from build123d import *

# Parameters (mm, degrees)
SKETCH1_R           = 14
SKETCH1_R_2         = 9
BOSS_EXTRUDE1_DEPTH = 17.5
SKETCH5_R           = 9.5
SKETCH5_R_2         = 7
BOSS_EXTRUDE2_DEPTH = 9.5
BOSS_EXTRUDE3_DEPTH = 2.5
SKETCH7_W           = 5
SKETCH7_H           = 17.5
BOSS_EXTRUDE4_DEPTH = 0.225023
BOSS_EXTRUDE5_DEPTH = 2.5
BOSS_EXTRUDE9_DEPTH = 2.5


with BuildPart() as part:
    # Sketch1 → Boss-Extrude1 (new, symmetric)
    with BuildSketch(Plane.XY):
        Circle(SKETCH1_R)
        Circle(SKETCH1_R_2, mode=Mode.SUBTRACT)
    extrude(amount=BOSS_EXTRUDE1_DEPTH, both=True)



with BuildPart() as body_2:
    # Sketch5 → Boss-Extrude2 (new, symmetric)
    with BuildSketch(Plane(origin=(0, 0, 0), x_dir=(0, 0, -1), z_dir=(1, 0, 0))):
        with Locations((0, 26)):
            Circle(SKETCH5_R)
        with Locations((0, 26)):
            Circle(SKETCH5_R_2, mode=Mode.SUBTRACT)
    extrude(amount=BOSS_EXTRUDE2_DEPTH, both=True)

    # Sketch6 → Boss-Extrude3 (add, symmetric)
    with BuildSketch(Plane(origin=(0, 0, 0), x_dir=(0, 0, -1), z_dir=(1, 0, 0))):
        with BuildLine():
            Line((-8.311766618, 30.600492984), (-17.5, 14))
            Line((-17.5, 14), (0, 14))
            Line((0, 14), (0, 16.5))
            ThreePointArc((0, 16.5), (-8.183968577, 21.175825633), (-8.311766618, 30.600492984))
        make_face()
    extrude(amount=BOSS_EXTRUDE3_DEPTH, both=True)


with BuildPart() as part_1:
    add(part.part)

    add(body_2.part)  # Boss-Extrude4 merges body 2
    # Sketch7 → Boss-Extrude4 (add)
    with BuildSketch(Plane.XZ.offset(-14)):
        with Locations((0, 8.75)):
            Rectangle(SKETCH7_W, SKETCH7_H)
    extrude(amount=BOSS_EXTRUDE4_DEPTH)

    # Sketch8 → Boss-Extrude5 (add, symmetric)
    with BuildSketch(Plane(origin=(0, 0, 0), x_dir=(0, 0, -1), z_dir=(1, 0, 0))):
        with BuildLine():
            Line((17.5, 14), (8.311766618, 30.600492984))
            ThreePointArc((8.311766618, 30.600492984), (9.198146087, 28.375733269), (9.5, 26))
            ThreePointArc((9.5, 26), (6.717514421, 19.282485579), (0, 16.5))
            Line((0, 16.5), (0, 14))
            Line((0, 14), (0, 13.650311759))
            Line((0, 13.650311759), (17.5, 13.650311759))
            Line((17.5, 13.650311759), (17.5, 14))
        make_face()
    extrude(amount=BOSS_EXTRUDE5_DEPTH, both=True)

    # Sketch9 → Boss-Extrude9 (add, symmetric)
    with BuildSketch(Plane.XY):
        with BuildLine():
            ThreePointArc((-13.359188152, 4.187134094), (-8.28794675, 11.283170594), (0, 14))
            Line((0, 14), (0, 16.5))
            Line((0, 16.5), (0, 17.5))
            Line((0, 17.5), (-9.5, 17.5))
            Line((-9.5, 17.5), (-9.5, 16.5))
            Line((-9.5, 16.5), (-13.359188152, 4.187134094))
        make_face()
    boss_extrude9 = extrude(amount=BOSS_EXTRUDE9_DEPTH, both=True)

    # Mirror9: Boss-Extrude9 across plane
    add(boss_extrude9.mirror(Plane(origin=(0, 0, 0), x_dir=(0, 0, 1), z_dir=(1, 0, 0))))


solid = part_1.part
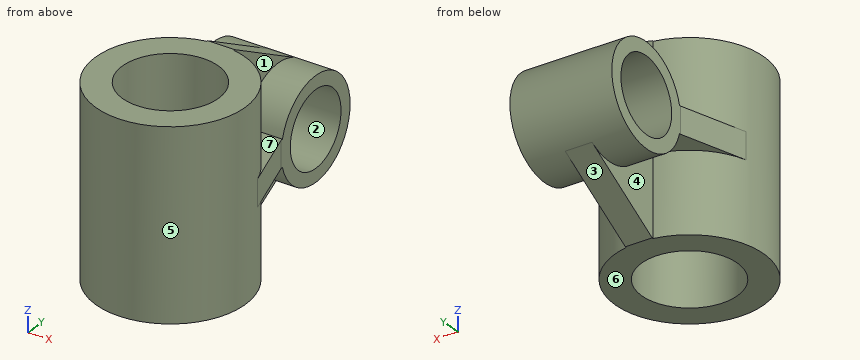
Can you work these out from the model? Positions are in its coordinate system, mm. Face numbers are marked on the shaded views. A direction names the side the tool comes from. Coordinates: 2 decimals unless noted, no trailing zeros. Order: outer loops, then holes, each group sorted by start corner. A loop starts at its lowest first (then second) coordinate and runs counter-clockwise, first axis right, second up. Notation, with made-up numbers: M 33.5,46.25 L 58.5,46.25 A18 ccw 58.5,66.25 Z; hole C 41,81 d3. An arc over 180 degrees is marked long. Answer as CSV lines item,"result".
(1) If we mould it in two halves opening along Z, with no side actions, what happens to the marked faces 1, 2 and 3? For each: released by +Z, released by -Z, zero draft, split by the parting line, or undercut.
Geometry check:
face 1,"zero draft"
face 2,"undercut"
face 3,"released by -Z"
(2) Suppose I cut it at C-C on x = 0. Please give me the cut outline in (y, z).
Geometry check:
outline,"M -14,-17.5 L -9,-17.5 L -9,17.5 L -14,17.5 Z; M 9,-17.5 L 14,-17.5 L 30.6,-8.31 A9.5 ccw 30.6,8.31 L 14,17.5 L 9,17.5 Z; hole C 26,0 d14"
(3) On a 3-axis mill with a long thin cutter (end or side, diameter ignored), from which of +Z, -Z, +X, -X, +Y, -Y can I reach the whole of each face in a straight line? I mean the marked faces 4, 5, 6 and 7. Say none if no direction works.
Geometry check:
face 4,"-Z, -X"
face 5,"none"
face 6,"-Z, +X, -X, +Y, -Y"
face 7,"+Z, +X"
(4) Suppose I cut it at A-A on y = 0. Please give me the cut outline in (x, z).
Geometry check:
outline,"M -14,-17.5 L -9,-17.5 L -9,17.5 L -14,17.5 Z; M 9,-17.5 L 14,-17.5 L 14,17.5 L 9,17.5 Z"
(5) Please list where these lines run through material, in increasing order: L1, parallel to Y at x = 6.5, z = -3.5; L2, parallel to Y at x = 6, z = -8.5; L3, parallel to X at y = 19, z = 4.
Geometry check:
L1,"-12.4 to -6.22, 6.22 to 12.4, 17.17 to 19.94, 32.06 to 34.83"
L2,"-12.65 to -6.71, 6.71 to 12.65, 21.76 to 30.24"
L3,"-9.5 to 9.5"
(6) Suppose I cut it at B-B on z = 0. Please give me the cut outline in (x, y).
Geometry check:
outline,"M -13.36,4.19 A14 ccw long 13.36,4.19 L 9.5,16.5 L 9.5,19 L -9.5,19 L -9.5,16.5 Z; M -9.5,33 L 9.5,33 L 9.5,35.5 L -9.5,35.5 Z; hole C 0,0 d18"
(7) Suppose I cut it at D-D on y = 25. Please give me the cut outline in (x, z).
Geometry check:
outline,"M -9.5,-9.45 L -2.5,-9.45 L -2.5,-11.41 L 2.5,-11.41 L 2.5,-9.45 L 9.5,-9.45 L 9.5,-6.93 L -9.5,-6.93 Z; M -9.5,6.93 L 9.5,6.93 L 9.5,9.45 L 2.5,9.45 L 2.5,11.41 L -2.5,11.41 L -2.5,9.45 L -9.5,9.45 Z"
(8) I'm going to push flat-ended pins straight in: pin 1 (12 mm diameter, centred on y = 24.5, z = -11.5, fed in from -X); pin 2 (12 mm diameter, centred on y = 24, z = -11, fed in from +X); pin 3 (8 mm diameter, centred on x = -4, y = 25.5, fed in from +Z). Where does each tip first touch, or does it pass through?
Geometry check:
pin 1,"x = -9.5"
pin 2,"x = 9.5"
pin 3,"z = 13.19"
